CAD build for the part. Positions are in the model's coordinates, mm. A direction names the side the tool comes from. Round coordinates to 2 decimals unless told otherwise and drop trailing zeros. Write each loop counter-clockwise with the first axis right and the second up, starting at its lowest first coordinate (ties: lowest second). Pieces come first, ordered by that corner, then holes. Notation, with made-up numbers: (88, 49.5) - (95, 49.5) arc R15 cw to (95, 54.5) - close; hole circle Ø9 at (19.5, 52). An arc over 180 degrees is marked (long way). Put each result on its own line as item: value. Start each with the question number.
Item 1: Cut at A-A (y = 483.5). Give the cut face in (x, z).
Item 2: 3-axis set-ups, long thin cutter, end or side, ignore diameter. For faces 5 (the flat face through (-4, 166, 9)), 6 (the flat face through (0, 526, 0)), 7 (the cylindrical face through (2.48, 454.84, 7.87)): which of +Z, -Z, +X, -X, +Y, -Y reach the whole face in a straight line?
Item 3: Mould opens along Y. For faces 1 (the flat face through (-4, 376, 9)), 2 (the cylindrical face through (-8.054, 92.072, -1.788)), 3 (the cylindrical face through (-0.867, 505.5, 3.905)), 4 (the flat face through (0, 0, 0)) say: released by +Y, released by -Y, zero draft, split by the parting line, or undercut.
Item 4: Cut at B-B (y = 385.5). Give the cut face in (x, z).
Item 5: Drill centre lines: line 1 (X direction, y = 130, z = 0); line 2 (Y direction, x = -5.75, z = -5); line 3 (Z direction, x = 1.25, y = 218.5). Where is each one in solid material? Low to high. Write a range as from..to.
Item 6: Pin check, flat tips, straight feed: pin 1 Ø5 at (x, z) = (3, -4) entering from -Y; pin 2 Ø1.5 at (y, z) = (221, 5.5) entering from +X; pin 3 Ø1 at (x, y) = (7.5, 297) entering from -Z; pin 4 Ø1.3 at (y, z) = (3, -5) entering from +X. Stop position of each tip, or through.
```python
from build123d import *

# Parameters (mm, degrees)
SKETCH1_R           = 8
BOSS_EXTRUDE1_DEPTH = 50
SKETCH2_R           = 8.25
BOSS_EXTRUDE2_DEPTH = 86
SKETCH3_R           = 8.5
BOSS_EXTRUDE3_DEPTH = 30
SKETCH4_R           = 10
BOSS_EXTRUDE4_DEPTH = 210
SKETCH5_R           = 8.5
BOSS_EXTRUDE5_DEPTH = 30
SKETCH6_R           = 8.25
BOSS_EXTRUDE6_DEPTH = 95
SKETCH32_R          = 8.25
BOSS_EXTRUDE7_DEPTH = 25
CUT_EXTRUDE1_START  = -3.2
CUT_EXTRUDE1_DEPTH  = 523.990079724
FILLET1_R           = 1


# Read off the part's stored shape, not the designer's step: M10x1.0 Machine Threads Stud1
with BuildPart() as part:
    # Sketch1 → Boss-Extrude1 (new body)
    with BuildSketch(Plane(origin=(0, 0, 0), x_dir=(1, 0, 0), z_dir=(0, 1, 0))):
        with Locations(Location((0, 0, 0), (0, 0, 270))):
            Circle(SKETCH1_R)
    extrude(amount=BOSS_EXTRUDE1_DEPTH)

    # Sketch2 → Boss-Extrude2 (add)
    with BuildSketch(Plane(origin=(0, 50, 0), x_dir=(1, 0, 0), z_dir=(0, 1, 0))):
        with Locations(Location((0, 0, 0), (0, 0, 270))):
            Circle(SKETCH2_R)
    extrude(amount=BOSS_EXTRUDE2_DEPTH)

    # Sketch3 → Boss-Extrude3 (add)
    with BuildSketch(Plane(origin=(0, 136, 0), x_dir=(1, 0, 0), z_dir=(0, 1, 0))):
        with Locations(Location((0, 0, 0), (0, 0, 270))):
            Circle(SKETCH3_R)
    extrude(amount=BOSS_EXTRUDE3_DEPTH)

    # Sketch4 → Boss-Extrude4 (add)
    with BuildSketch(Plane(origin=(0, 166, 0), x_dir=(1, 0, 0), z_dir=(0, 1, 0))):
        with Locations(Location((0, 0, 0), (0, 0, 270))):
            Circle(SKETCH4_R)
    extrude(amount=BOSS_EXTRUDE4_DEPTH)

    # Sketch5 → Boss-Extrude5 (add)
    with BuildSketch(Plane(origin=(0, 376, 0), x_dir=(1, 0, 0), z_dir=(0, 1, 0))):
        with Locations(Location((0, 0, 0), (0, 0, 270))):
            Circle(SKETCH5_R)
    extrude(amount=BOSS_EXTRUDE5_DEPTH)

    # Sketch6 → Boss-Extrude6 (add)
    with BuildSketch(Plane(origin=(0, 406, 0), x_dir=(1, 0, 0), z_dir=(0, 1, 0))):
        with Locations(Location((0, 0, 0), (0, 0, 270))):
            Circle(SKETCH6_R)
    extrude(amount=BOSS_EXTRUDE6_DEPTH)

    # Sketch32 → Boss-Extrude7 (add)
    with BuildSketch(Plane(origin=(0, 501, 0), x_dir=(1, 0, 0), z_dir=(0, 1, 0))):
        with Locations(Location((0, 0, 0), (0, 0, 270))):
            Circle(SKETCH32_R)
    extrude(amount=BOSS_EXTRUDE7_DEPTH)

    # M10x1.0 Machine Threads Stud1 outline → M10x1.0 Machine Threads Stud1 (revolve, cut)
    with BuildSketch(Plane.XY):
        with BuildLine():
            Line((8.25, 526), (4.4455, 526))
            Line((4.4455, 526), (5, 525.4455))
            Line((5, 525.4455), (5, 508))
            Line((5, 508), (4.066987298, 506.383974596))
            ThreePointArc((4.066987298, 506.383974596), (4.017037087, 506.263384119), (4, 506.133974596))
            Line((4, 506.133974596), (4, 504.883974596))
            ThreePointArc((4, 504.883974596), (4.14644661, 504.530421205), (4.5, 504.383974596))
            Line((4.5, 504.383974596), (8.25, 504.383974596))
            Line((8.25, 504.383974596), (8.25, 526))
        make_face()
    revolve(axis=Axis((0, 0, 0), (0, 1, 0)), mode=Mode.SUBTRACT)

    # Sketch34 → Cut-Extrude1 (cut, through all)
    with BuildSketch(Plane.XY.offset(CUT_EXTRUDE1_START)):
        with BuildLine():
            Line((3, -11), (-3, -11))
            Line((-3, -11), (-3, 11))
            ThreePointArc((-3, 11), (0, 14), (3, 11))
            Line((3, 11), (3, -11))
        make_face()
    extrude(amount=-CUT_EXTRUDE1_DEPTH, mode=Mode.SUBTRACT)

    # Fillet1
    # the kernel refuses this fillet: 1 mm, written as the material it adds along each edge
    with BuildSketch(Plane(origin=(0, 376, 0), x_dir=(0, 0, 1), z_dir=(-1, 0, 0))) as fillet1_piece_1:
        with BuildLine():
            CenterArc((8.5 + FILLET1_R, FILLET1_R), FILLET1_R, 180, 90)
            Line((8.5, FILLET1_R), (8.5 - FILLET1_R * 0.02, FILLET1_R))
            Line((8.5 - FILLET1_R * 0.02, FILLET1_R), (8.5 - FILLET1_R * 0.02, -FILLET1_R * 0.02))
            Line((8.5 - FILLET1_R * 0.02, -FILLET1_R * 0.02), (8.5 + FILLET1_R, -FILLET1_R * 0.02))
            Line((8.5 + FILLET1_R, -FILLET1_R * 0.02), (8.5 + FILLET1_R, 0))
        make_face()
    revolve(axis=Axis((0, 376, 0), (0, 1, 0)))
    with BuildSketch(Plane(origin=(0, 406, 0), x_dir=(0, 0, 1), z_dir=(-1, 0, 0))) as fillet1_piece_2:
        with BuildLine():
            CenterArc((9.25, 0.661437828), FILLET1_R, 180, 41.409622109)
            Line((8.25, 0.661437828), (8.23, 0.661437828))
            Line((8.23, 0.661437828), (8.23, 0))
            Line((8.23, 0), (8.25, -0.02))
            ThreePointArc((8.25, -0.02), (8.375, -0.02), (8.485, -0.013228757))
            Line((8.485, -0.013228757), (8.5, 0))
        make_face()
    revolve(axis=Axis((0, 406, 0), (0, 1, 0)))
    with BuildSketch(Plane(origin=(0, 50, 0), x_dir=(0, 0, 1), z_dir=(-1, 0, 0))) as fillet1_piece_3:
        with BuildLine():
            CenterArc((9, -0.661437828), FILLET1_R, 138.590377891, 41.409622109)
            Line((8, -0.661437828), (7.98, -0.661437828))
            Line((7.98, -0.661437828), (7.98, 0))
            Line((7.98, 0), (8, 0.02))
            ThreePointArc((8, 0.02), (8.125, 0.02), (8.235, 0.013228757))
            Line((8.235, 0.013228757), (8.25, 0))
        make_face()
    revolve(axis=Axis((0, 50, 0), (0, 1, 0)))
    with BuildSketch(Plane(origin=(0, 136, 0), x_dir=(0, 0, 1), z_dir=(-1, 0, 0))) as fillet1_piece_4:
        with BuildLine():
            CenterArc((9.25, -0.661437828), FILLET1_R, 138.590377891, 41.409622109)
            Line((8.25, -0.661437828), (8.23, -0.661437828))
            Line((8.23, -0.661437828), (8.23, 0))
            Line((8.23, 0), (8.25, 0.02))
            ThreePointArc((8.25, 0.02), (8.375, 0.02), (8.485, 0.013228757))
            Line((8.485, 0.013228757), (8.5, 0))
        make_face()
    revolve(axis=Axis((0, 136, 0), (0, 1, 0)))
    with BuildSketch(Plane(origin=(0, 166, 0), x_dir=(0, 0, 1), z_dir=(-1, 0, 0))) as fillet1_piece_5:
        with BuildLine():
            CenterArc((8.5 + FILLET1_R, -FILLET1_R), FILLET1_R, 90, 90)
            Line((8.5, -FILLET1_R), (8.5 - FILLET1_R * 0.02, -FILLET1_R))
            Line((8.5 - FILLET1_R * 0.02, -FILLET1_R), (8.5 - FILLET1_R * 0.02, FILLET1_R * 0.02))
            Line((8.5 - FILLET1_R * 0.02, FILLET1_R * 0.02), (8.5 + FILLET1_R, FILLET1_R * 0.02))
            Line((8.5 + FILLET1_R, FILLET1_R * 0.02), (8.5 + FILLET1_R, 0))
        make_face()
    revolve(axis=Axis((0, 166, 0), (0, 1, 0)))


solid = part.part
```
Output values:
1. outline: circle Ø16.5 at (0, 0)
2. face 5: -Y
2. face 6: +Z, -Z, +X, -X, +Y
2. face 7: +Y
3. face 1: released by +Y
3. face 2: zero draft
3. face 3: undercut
3. face 4: released by -Y
4. outline: circle Ø17 at (0, 0)
5. line 1: -8.25..8.25
5. line 2: 0..504.38
5. line 3: -9.92..9.92
6. pin 1: y = 0
6. pin 2: x = 8.8
6. pin 3: z = -7.14
6. pin 4: x = 6.71
